Here's the drawing with two shaded views (mm, measured from the low corner). I have some questions. Coordinates: 2 decimals unless noted, no trailing zeros. Loops run counter-clockwise (first coordinate to the right, second up) from the corner with the lowest first, then second, coordinate; pieces in that order, holes last.
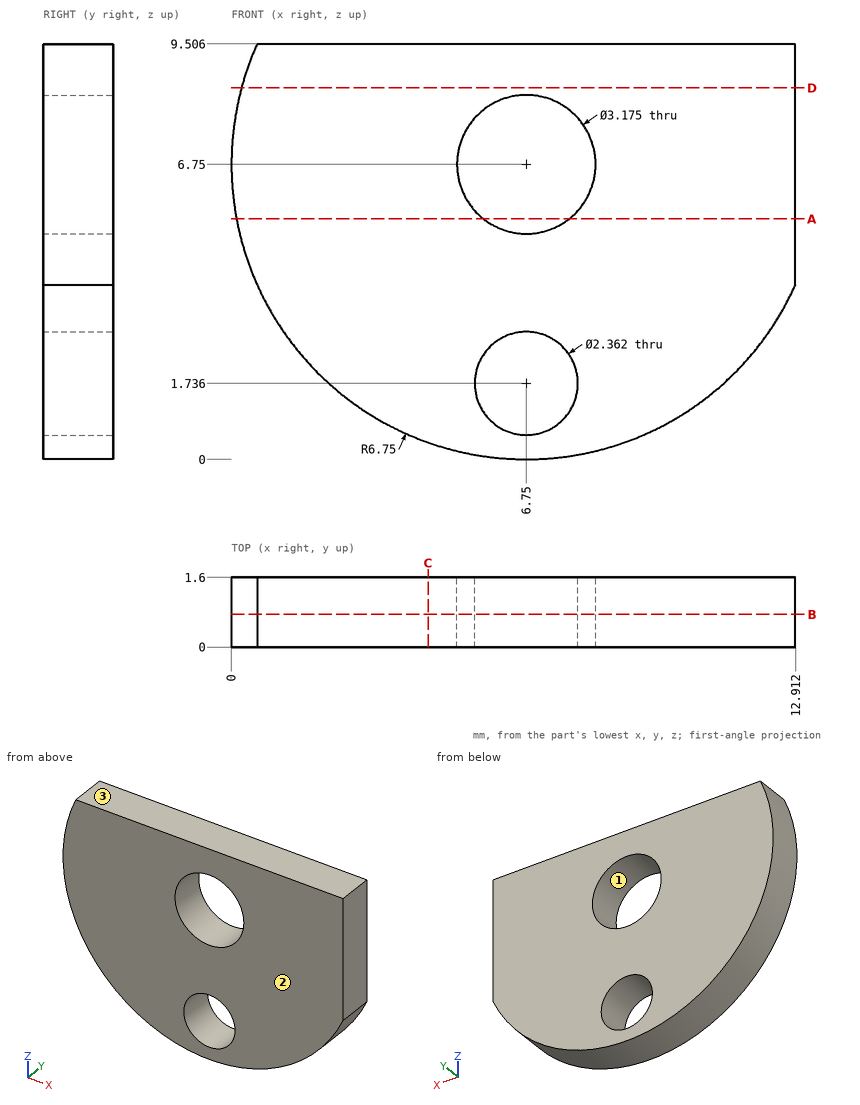
(1) If I drill on probe 1 along Z at (x, y) = (6.25, 0.25) (1 decimal); probe 2 along Z at (x, y) = (6.5, 0.4) (1 decimal); probe 3 along X at (y, z) = (1.4, 4) (1 decimal), over which ranges is the centre line in solid material (lowest first)?
Check values:
probe 1: z = 0 to 0.7, 2.8 to 5.2, 8.3 to 9.5
probe 2: z = 0 to 0.6, 2.9 to 5.2, 8.3 to 9.5
probe 3: x = 0.6 to 12.9
(2) If we mould it in two halves opening along Z, with no side actions, what happens to the marked faces 1, 2 and 3? For each: released by +Z, released by -Z, zero draft, split by the parting line, or undercut.
Check values:
face 1: undercut
face 2: zero draft
face 3: released by +Z
(3) I want a section at C-C on x = 4.5. Write out the boundary of the cut face in (y, z) (1 decimal).
Check values:
outline: (0, 0.4) - (1.6, 0.4) - (1.6, 9.5) - (0, 9.5) - close
(4) I want a section at A-A on z = 5.5. Write out the boundary of the cut face in (x, y).
Check values:
outline: (0.12, 0) - (5.77, 0) - (5.77, 1.6) - (0.12, 1.6) - close; (7.73, 0) - (12.91, 0) - (12.91, 1.6) - (7.73, 1.6) - close
(5) I want a section at D-D on z = 8.5. Write out the boundary of the cut face in (x, y).
Check values:
outline: (0.23, 0) - (12.91, 0) - (12.91, 1.6) - (0.23, 1.6) - close
(6) I want a section at B-B on y = 0.75. State how many separate pieces and enclosed holes the cut face has.
Check values:
separate pieces: 1
enclosed holes: 2
